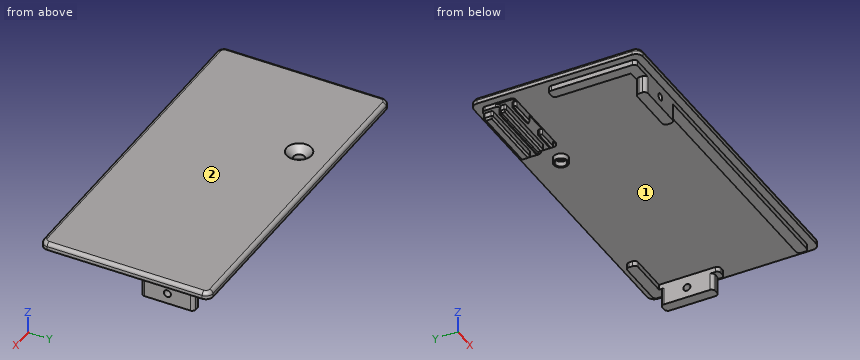
from build123d import *

# Parameters (mm, degrees)
SKETCH027_W     = 95
SKETCH027_H     = 48
PAD011_DEPTH    = 2
SKETCH028_R     = 2
PAD012_DEPTH    = 1.5
SKETCH032_W     = 22.9
SKETCH032_H     = 4.9
PAD013_DEPTH    = 1.2
SKETCH033_W     = 22.9
SKETCH033_H     = 4.3
PAD014_DEPTH    = 0.4
SKETCH034_W     = 15
SKETCH034_H     = 3
SKETCH034_W_2   = 3
SKETCH034_H_2   = 15
PAD015_DEPTH    = 5
SKETCH035_R     = 1
POCKET015_DEPTH = 5
SKETCH036_R     = 1
POCKET016_DEPTH = 5
SKETCH037_R     = 1.55
POCKET017_DEPTH = 7
FILLET_R        = 2
FILLET001_R     = 1
CHAMFER_SIZE    = 2
FILLET002_R     = 1
SKETCH047_W     = 20
SKETCH047_H     = 1.15
SKETCH047_H_2   = 1.4
PAD020_DEPTH    = 2
SKETCH048_W     = 20
SKETCH048_H     = 2.6
SKETCH048_H_2   = 0.6
PAD021_DEPTH    = 2
FILLET012_R     = 0.5
CHAMFER005_SIZE = 0.5
CHAMFER006_SIZE = 0.5
SKETCH051_W     = 6
SKETCH051_H     = 1.15
POCKET022_DEPTH = 2
FILLET015_R     = 0.5


with BuildPart() as part:
    # Sketch027 → Pad011 (new body)
    with BuildSketch(Plane.XY):
        with Locations((47.5, -34)):
            Rectangle(SKETCH027_W, SKETCH027_H)
    extrude(amount=PAD011_DEPTH)

    # Sketch028 (on Face5 of Pad011) → Pad012 (join)
    with BuildSketch(Plane(origin=(0, 0, 0), x_dir=(1, 0, 0), z_dir=(0, 0, -1))):
        with Locations((30.5, 19.3)):
            Circle(SKETCH028_R)
        Polygon((2.1, 30.9), (5.1, 30.9), (5.1, 52.9), (92.9, 52.9), (92.9, 55.9), (2.1, 55.9), align=None)
        Polygon((89.9, 32.1), (92.9, 32.1), (92.9, 12.1), (77.9, 12.1), (77.9, 15.1), (89.9, 15.1), align=None)
    extrude(amount=PAD012_DEPTH)

    # Sketch032 (on Face4 of Pad012) → Pad013 (join)
    with BuildSketch(Plane(origin=(0, 0, 0), x_dir=(1, 0, 0), z_dir=(0, 0, -1))):
        with Locations((13.55, 14.55)):
            Rectangle(SKETCH032_W, SKETCH032_H)
    extrude(amount=PAD013_DEPTH)

    # Sketch033 (on Face4 of Pad013) → Pad014 (join)
    with BuildSketch(Plane(origin=(0, 0, 0), x_dir=(1, 0, 0), z_dir=(0, 0, -1))):
        with Locations((13.55, 19.15)):
            Rectangle(SKETCH033_W, SKETCH033_H)
    extrude(amount=PAD014_DEPTH)

    # Sketch034 (on Face26 of Pad014) → Pad015 (join)
    with BuildSketch(Plane(origin=(0, 0, -1.5), x_dir=(1, 0, 0), z_dir=(0, 0, -1))):
        with Locations((15, 54.4)):
            Rectangle(SKETCH034_W, SKETCH034_H)
        with Locations((91.4, 23)):
            Rectangle(SKETCH034_W_2, SKETCH034_H_2)
    extrude(amount=PAD015_DEPTH)

    # Sketch035 (on Face33 of Pad015) → Pocket015 (cut)
    with BuildSketch(Plane.YZ.offset(92.9)):
        with Locations((-23, -3.5)):
            Circle(SKETCH035_R)
    extrude(amount=-POCKET015_DEPTH, mode=Mode.SUBTRACT)

    # Sketch036 (on Face28 of Pocket015) → Pocket016 (cut)
    with BuildSketch(Plane.XZ.offset(55.9)):
        with Locations((15, -3.5)):
            Circle(SKETCH036_R)
    extrude(amount=-POCKET016_DEPTH, mode=Mode.SUBTRACT)

    # Sketch037 (on Face34 of Pocket016) → Pocket017 (cut)
    with BuildSketch(Plane(origin=(0, 0, -1.5), x_dir=(1, 0, 0), z_dir=(0, 0, -1))):
        with Locations((30.5, 19.3)):
            Circle(SKETCH037_R)
    extrude(amount=-POCKET017_DEPTH, mode=Mode.SUBTRACT)

    # Fillet
    fillet_edges = [part.edges().sort_by_distance(p)[0] for p in [
        (0, -58, 1),
        (0, -10, 1),
        (95, -58, 1),
        (95, -10, 1),
    ]]
    fillet(fillet_edges, radius=FILLET_R)

    # Fillet001
    fillet001_edges = [part.edges().sort_by_distance(p)[0] for p in [
        (47.5, -58, 2),
    ]]
    fillet(fillet001_edges, radius=FILLET001_R)

    # Chamfer
    chamfer_edges = [part.edges().sort_by_distance(p)[0] for p in [
        (28.95, -19.3, 2),
    ]]
    chamfer(chamfer_edges, length=CHAMFER_SIZE)

    # Fillet002
    fillet002_edges = [part.edges().sort_by_distance(p)[0] for p in [
        (2.1, -30.9, -0.75),
        (5.1, -30.9, -0.75),
        (2.1, -21.3, -0.2),
        (2.1, -17, -0.8),
        (2.1, -12.1, -0.6),
        (25, -12.1, -0.6),
        (25, -17, -0.8),
        (25, -21.3, -0.2),
        (92.9, -55.9, -0.75),
        (92.9, -52.9, -0.75),
        (92.9, -32.1, -0.75),
        (92.9, -12.1, -0.75),
        (77.9, -12.1, -0.75),
        (92.9, -15.5, -4),
        (89.9, -15.5, -4),
        (92.9, -30.5, -4),
        (89.9, -32.1, -0.75),
        (89.9, -30.5, -4),
        (77.9, -15.1, -0.75),
        (22.5, -55.9, -4),
        (7.5, -55.9, -4),
        (2.1, -55.9, -0.75),
        (7.5, -52.9, -4),
        (22.5, -52.9, -4),
    ]]
    fillet(fillet002_edges, radius=FILLET002_R)

    # Sketch047 (on Face61 of Fillet002) → Pad020 (join)
    with BuildSketch(Plane(origin=(0, 0, -0.4), x_dir=(1, 0, 0), z_dir=(0, 0, -1))):
        with Locations((13.1, 20.725)):
            Rectangle(SKETCH047_W, SKETCH047_H)
        with Locations((13.1, 17.7)):
            Rectangle(SKETCH047_W, SKETCH047_H_2)
    extrude(amount=PAD020_DEPTH)

    # Sketch048 (on Face60 of Pad020) → Pad021 (join)
    with BuildSketch(Plane(origin=(0, 0, -1.2), x_dir=(1, 0, 0), z_dir=(0, 0, -1))):
        with Locations((13.1, 13.4)):
            Rectangle(SKETCH048_W, SKETCH048_H)
        with Locations((13.1, 16.7)):
            Rectangle(SKETCH048_W, SKETCH048_H_2)
    extrude(amount=PAD021_DEPTH)

    # Fillet012
    fillet012_edges = [part.edges().sort_by_distance(p)[0] for p in [
        (3.1, -21.3, -1.4),
        (3.1, -20.15, -1.4),
        (3.1, -18.4, -1.4),
        (23.1, -21.3, -1.4),
        (23.1, -20.15, -1.4),
        (23.1, -18.4, -1.4),
        (23.1, -14.7, -2.2),
        (23.1, -16.4, -2.2),
        (3.1, -16.4, -2.2),
        (3.1, -14.7, -2.2),
        (23.1, -12.1, -2.2),
        (3.1, -12.1, -2.2),
    ]]
    fillet(fillet012_edges, radius=FILLET012_R)

    # Chamfer005
    chamfer005_edges = [part.edges().sort_by_distance(p)[0] for p in [
        (13.1, -16.4, -3.2),
    ]]
    chamfer(chamfer005_edges, length=CHAMFER005_SIZE)

    # Chamfer006
    chamfer006_edges = [part.edges().sort_by_distance(p)[0] for p in [
        (13.1, -14.7, -3.2),
        (13.1, -18.4, -2.4),
        (13.1, -20.15, -2.4),
    ]]
    chamfer(chamfer006_edges, length=CHAMFER006_SIZE)

    # Sketch051 (on Face70 of Chamfer006) → Pocket022 (cut)
    with BuildSketch(Plane(origin=(0, 0, -2.4), x_dir=(1, 0, 0), z_dir=(0, 0, -1))):
        with Locations((13.6, 20.725)):
            Rectangle(SKETCH051_W, SKETCH051_H)
    extrude(amount=-POCKET022_DEPTH, mode=Mode.SUBTRACT)

    # Fillet015
    fillet015_edges = [part.edges().sort_by_distance(p)[0] for p in [
        (10.6, -20.15, -1.15),
        (10.6, -21.3, -1.15),
        (16.6, -20.15, -1.15),
        (16.6, -21.3, -1.15),
    ]]
    fillet(fillet015_edges, radius=FILLET015_R)


solid = part.part
Source: CAD feature listing. Evaluate the final solid. Frame: model axes, mm. Face numbers are marked on the shaded views. Coordinates: 2 decimals unless noted, no trailing zeros. Loops run counter-clockwise (first coordinate to the right, second up) from the corner with the lowest first, then second, coordinate; pieces in that order, holes last. Notation, with made-up numbers: (37.5, 88.25) - (46.5, 88.25) arc R26 cw to (46.5, 110.25) - close; hole circle Ø10 at (13, 69.5). An arc over 180 degrees is marked (long way). One line per item, written item: value. Start each with the question number.
1. Mould query, pull axis X, two halves, no side actions, for the marked faces 1 and 2. Classes: pulls with the +X half, pulls with the -X half, needs draft (parallel to the pull), parting line crosses it, or undercut.
2. Ray query, L1, parallel to Y at x = 30.5, z = -0.4; L2, parallel to X at y = -19.3, z = -0.7; L3, parallel to X at y = -22.5, z = -2. Return the intervals inside material, ascending.
3. Contact query for flat-ended pins moving along their axis: P1, Ø1.9, axis at x = 4, y = -40, coming from the -Z side; P2, Ø1.5, axis at x = 58, y = -41.5, coming from the -Z side; P3, Ø0.5, axis at y = -13.5, z = -0.5, coming from the -X side; P4, Ø3, axis at x = 91.5, y = -31, coming from the -Z side. Output: stop coordinate, or through.
4. Section C-C (x = 30.5). Return the cut outline in (y, z), and give its area (3 significant figures).
5. Section D-D (x = 67.5). Return the cut outline in (y, z), and give its area (3 significant figures).
6. Section B-B (y = -40). Return the cut outline in (x, z).
Verdict:
1. face 1: undercut
1. face 2: needs draft
2. L1: y = -55.9 to -52.9, -21.3 to -20.85, -17.75 to -17.3
2. L2: x = 28.5 to 28.95, 32.05 to 32.5, 89.9 to 92.9
2. L3: x = 89.9 to 92.9
3. P1: stops at z = -1.5
3. P2: stops at z = 0
3. P3: stops at x = 2.1
3. P4: stops at z = -6.5
4. outline: (-58, 0) - (-55.9, 0) - (-55.9, -1.5) - (-52.9, -1.5) - (-52.9, 0) - (-21.3, 0) - (-21.3, -1.5) - (-20.85, -1.5) - (-20.85, 0) - (-22.85, 2) - (-57, 2) arc R1 ccw to (-58, 1) - close; (-17.75, -1.5) - (-17.3, -1.5) - (-17.3, 0) - (-10, 0) - (-10, 1) arc R1 ccw to (-11, 2) - (-15.75, 2) - (-17.75, 0) - close
4. area: 91.2 mm2
5. outline: (-58, 0) - (-55.9, 0) - (-55.9, -1.5) - (-52.9, -1.5) - (-52.9, 0) - (-10, 0) - (-10, 1) arc R1 ccw to (-11, 2) - (-57, 2) arc R1 ccw to (-58, 1) - close
5. area: 100 mm2
6. outline: (0, 0) - (2.1, 0) - (2.1, -1.5) - (5.1, -1.5) - (5.1, 0) - (95, 0) - (95, 1) arc R1 ccw to (94, 2) - (1, 2) arc R1 ccw to (0, 1) - close
